For this review, use the dimensioned drawing (mm, ordinates from the lowest corner) and the shaded views. A direction names the side the tool comes from. Give positions to 0.01 mm unless a question says otherwise; leave off trailing zeros. Write each loop counter-clockwise with the first axis right and the second up, starting at its lowest first coordinate (ties: lowest second). Pieces come first, ordered by that corner, then holes.
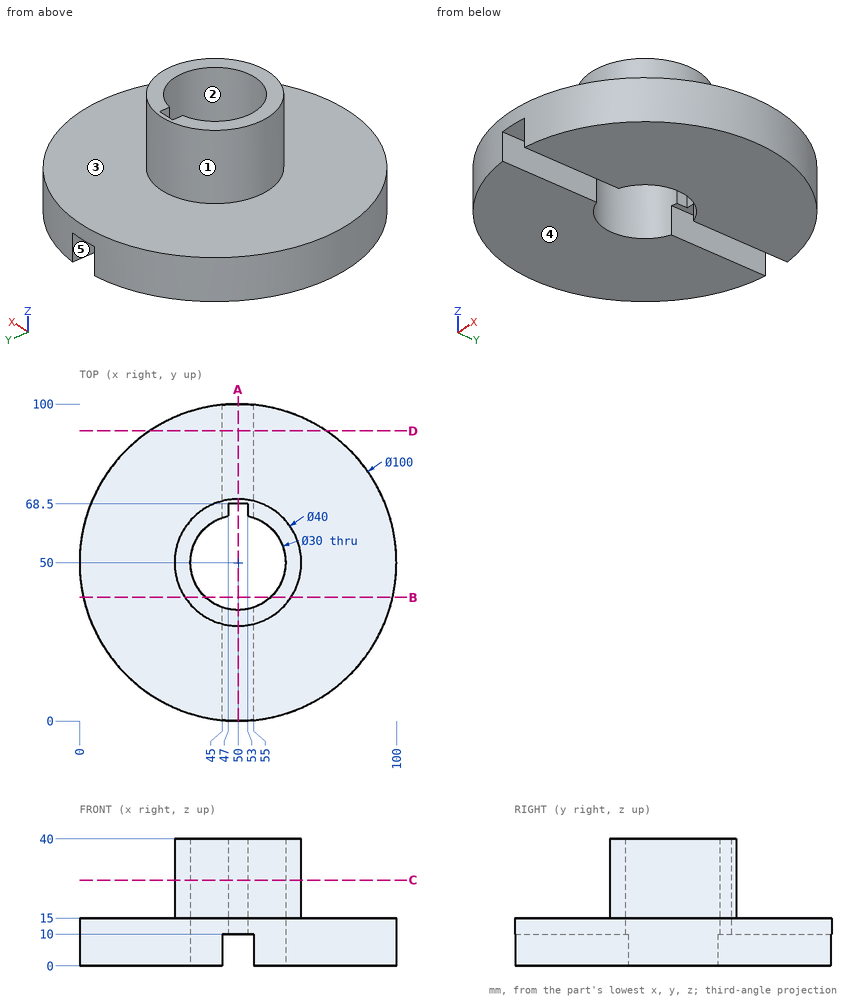
(1) We need section D-D (y = 91.5). Write out the cut boundary in (x, z), and give its area (3 significant figures).
(2) For L1, parallel to X at y = 50, z = 9; L2, parallel to Y at x = 50, z = 29; L3, parallel to Z at x = 41, y = 79, list the stretches that pass through material, from the lowest coordinate up.
(3) Tool access review of the marked faces 4 and 5: name each direction out of +Z, -Z, +X, -X, +Y, -Y from which nothing blocks a thin tool from reaching the whole face with its end or side.
(4) Clearance check with flat-ended pins moving along their axes: pin 1 Ø3 at (y, z) = (87, 6.5) entering from -X; pin 2 Ø4 at (y, z) = (41.5, 24.5) entering from -X; pin 3 Ø1 at (y, z) = (55.5, 21) entering from -X; pin 4 Ø4 at (y, z) = (51, 12.5) entering from +X. State where each tip first meets the part, or that it passes through.
(5) We need section C-C (z = 27). Write out the cut boundary in (x, y), and give its area (3 significant figures).
(6) We need section A-A (x = 50). Write out the cut boundary in (y, z), and give its area (3 significant figures).
(7) The part is to be moulded in two halves that separate along X. For the marked faces 1, 2 and 3, say which applies: +X half, -X half, draft (parallel to the pull), parting line (faces both ways), or undercut.
(8) We need section B-B (y = 39). Write out the cut boundary in (x, z) (3 decimals), and give its area (3 significant figures).
The answers:
1. outline: (22.11, 0) - (45, 0) - (45, 10) - (55, 10) - (55, 0) - (77.89, 0) - (77.89, 15) - (22.11, 15) - close
1. area: 737 mm2
2. L1: x = 0 to 35, 65 to 100
2. L2: y = 30 to 35, 68.5 to 70
2. L3: z = 0 to 15
3. face 4: -Z, +X, -X, +Y, -Y
3. face 5: -Z, +Y, -Y
4. pin 1: stops at x = 14.79
4. pin 2: stops at x = 31.09
4. pin 3: stops at x = 30.64
4. pin 4: stops at x = 100
5. outline: circle Ø40 at (50, 50); hole (47, 64.7) arc R15 ccw (long way) to (53, 64.7) - (53, 68.5) - (47, 68.5) - close
5. area: 528 mm2
6. outline: (0, 10) - (35, 10) - (35, 40) - (30, 40) - (30, 15) - (0, 15) - close; (68.5, 10) - (100, 10) - (100, 15) - (70, 15) - (70, 40) - (68.5, 40) - close
6. area: 495 mm2
7. face 1: parting line
7. face 2: undercut
7. face 3: draft
8. outline: (1.225, 0) - (39.802, 0) - (39.802, 40) - (33.297, 40) - (33.297, 15) - (1.225, 15) - close; (60.198, 0) - (98.775, 0) - (98.775, 15) - (66.703, 15) - (66.703, 40) - (60.198, 40) - close
8. area: 1,480 mm2
